```python
from build123d import *

# Parameters (mm, degrees)
GUARD_BASE_R     = 37.5
GUARD_DEPTH      = 5
AXLE_HOLE_BASE_R = 26.25
AXLE_HOLE_DEPTH  = 6


with BuildPart() as part:
    # Guard base → Guard (new body)
    with BuildSketch(Plane.XY):
        Circle(GUARD_BASE_R)
    extrude(amount=GUARD_DEPTH)

    # Axle hole base → Axle hole (cut, through all)
    with BuildSketch(Plane.XY.offset(5)):
        Circle(AXLE_HOLE_BASE_R)
    extrude(amount=-AXLE_HOLE_DEPTH, mode=Mode.SUBTRACT)

    # Mate ring room base → Mate ring room (revolve, cut)
    with BuildSketch(Plane(origin=(0, 0, 0), x_dir=(1, 0, 0), z_dir=(0, 1, 0))):
        Polygon((26.25, -5), (27, -5), (26.25, -4.25), align=None)
        Polygon((26.25, 0), (27, 0), (26.25, -0.75), align=None)
    revolve(axis=Axis((0, 0, 0), (0, 0, -1)), mode=Mode.SUBTRACT)


solid = part.part
```
Work out the finished part from the listing and answer in its coordinate system (mm). Coordinates: 2 decimals unless noted, no trailing zeros. Loops run counter-clockwise (first coordinate to the right, second up) from the corner with the lowest first, then second, coordinate; pieces in that order, holes last. Notation, with made-up numbers: M 89.25,13.5 L 117.25,13.5 A14 ccw 117.25,25.5 Z; hole C -3,-30 d9. An arc over 180 degrees is marked long. Use CSV: the item, a comma, the result in double quotes. Start each with the question number.
(1) Given pin 1 Ø1 at (y, z) = (-15, 0.5) entering from +X, flat-ended and moving along its own axis, determine where the tip first touches the part or whether it passes through.
(2) Find section A-A, the plane y = 0. Give the vertices of the cut face in (x, z), then the cut area to 3 significant figures.
(3) For a pull along X with two mould halves and no side action, classify faces 1 (the face through (-4.88, 37.18, 2.46)), 2 (the face through (25, 8, 3)), 3 (the face through (-26, 9, 0)) as +X half, -X half, draft (parallel to the pull), parting line (faces both ways), or undercut.
(4) Find section C-C, the plane z = 1.8. Give the vertices of the cut face in (x, y).
(5) Consider line 1 (Y direction, x = 0, z = 1.65); line 2 (X direction, y = 4, z = 1.65); line 3 (Y direction, x = 22, z = 0.85). Determine where each line is inside the solid, lowest interval first.
(6) Find section D-D, the plane x = 30. Give the vertices of the cut face in (y, z), then the cut area to 3 significant figures.
Recorded:
1,pin 1,"stops at x = 34.58"
2,outline,"M -37.5,0 L -27,0 L -26.25,0.75 L -26.25,4.25 L -27,5 L -37.5,5 Z; M 26.25,0.75 L 27,0 L 37.5,0 L 37.5,5 L 27,5 L 26.25,4.25 Z"
2,area,"111 mm^2"
3,face 1,"parting line"
3,face 2,"undercut"
3,face 3,"draft"
4,outline,"C 0,0 d75; hole C 0,0 d52.5"
5,line 1,"y = -37.5 to -26.25, 26.25 to 37.5"
5,line 2,"x = -37.29 to -25.94, 25.94 to 37.29"
5,line 3,"y = -30.37 to -14.32, 14.32 to 30.37"
6,outline,"M -22.5,0 L 22.5,0 L 22.5,5 L -22.5,5 Z"
6,area,"225 mm^2"
